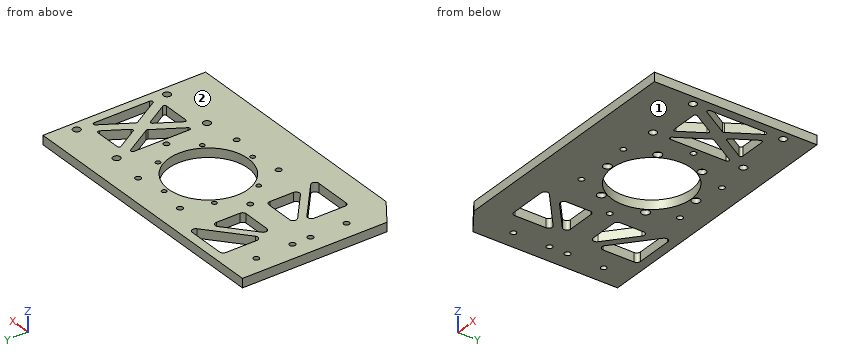
from build123d import *

# Parameters (mm, degrees)
SKETCH_1_W             = 150
SKETCH_1_H             = 80
SKETCH_1_R             = 1.3
SKETCH_1_R_2           = 22
EXTRUDE_1_DEPTH        = 5
SKETCH_3_R             = 1.55
SKETCH_3_R_2           = 1.582849294
CUT_EXTRUDE_3_DEPTH    = 12.5
CUT_EXTRUDE_5_DEPTH    = 8
FILLET_3_R             = 2
FILLET_3_OF_MIRROR_2_R = 2
EXTRUDE_4_DEPTH        = 5
FILLET_5_R             = 5
SKETCH_11_R            = 1.55
CUT_EXTRUDE_7_DEPTH    = 25
SKETCH_12_R            = 2.05
CUT_EXTRUDE_8_DEPTH    = 10
CUT_EXTRUDE_9_DEPTH    = 10
FILLET_6_R             = 1
EXTRUDE_5_DEPTH        = 5
SKETCH_16_R            = 2.25
CUT_EXTRUDE_10_DEPTH   = 2.5
CUT_EXTRUDE_START      = -10
CUT_EXTRUDE_11_DEPTH   = 10


with BuildPart() as part:
    # 草图1 → 凸台-拉伸1 (new body)
    with BuildSketch(Plane.XY):
        with Locations((-5, 0)):
            Rectangle(SKETCH_1_W, SKETCH_1_H)
        with Locations((0, -24.5)):
            Circle(SKETCH_1_R, mode=Mode.SUBTRACT)
        with Locations((-21.217622393, -12.25)):
            Circle(SKETCH_1_R, mode=Mode.SUBTRACT)
        with Locations((-21.217622393, 12.25)):
            Circle(SKETCH_1_R, mode=Mode.SUBTRACT)
        Circle(SKETCH_1_R_2, mode=Mode.SUBTRACT)
        with Locations((0, 24.5)):
            Circle(SKETCH_1_R, mode=Mode.SUBTRACT)
        with Locations((21.217622393, 12.25)):
            Circle(SKETCH_1_R, mode=Mode.SUBTRACT)
        with Locations((21.217622393, -12.25)):
            Circle(SKETCH_1_R, mode=Mode.SUBTRACT)
    extrude(amount=EXTRUDE_1_DEPTH)

    # 草图3 → 切除-拉伸3 (cut)
    with BuildSketch(Plane.XY.offset(5)):
        with Locations((-70, -25)):
            Circle(SKETCH_3_R)
        with Locations((-70, -5)):
            Circle(SKETCH_3_R_2)
        with Locations((-70, 25)):
            Circle(SKETCH_3_R)
        with Locations((-70, 5)):
            Circle(SKETCH_3_R_2)
    extrude(amount=-CUT_EXTRUDE_3_DEPTH, mode=Mode.SUBTRACT)

    # 草图4 → 切除-拉伸5 (cut)
    with BuildSketch(Plane.XY.offset(5)):
        Polygon((-58, 35), (-30, 35), (-58, 11.505210327), align=None)
        Polygon((-35, 25.582872687), (-58, 6.28358117), (-35, 6.28358117), align=None)
    cut_extrude_5 = extrude(amount=-CUT_EXTRUDE_5_DEPTH, mode=Mode.SUBTRACT)

    # 圆角3
    fillet_3_edges = [part.edges().sort_by_distance(p)[0] for p in [
        (-35, 6.28358117, 2.5),
        (-58, 6.28358117, 2.5),
        (-35, 25.582872687, 2.5),
        (-30, 35, 2.5),
        (-58, 11.505210327, 2.5),
        (-58, 35, 2.5),
    ]]
    fillet(fillet_3_edges, radius=FILLET_3_R)

    # 镜向2: 切除-拉伸5 across plane
    add(cut_extrude_5.mirror(Plane.ZX), mode=Mode.SUBTRACT)

    # 圆角3 of 镜向2
    fillet_3_of_mirror_2_edges = [part.edges().sort_by_distance(p)[0] for p in [
        (-35, -6.28358117, 2.5),
        (-58, -6.28358117, 2.5),
        (-35, -25.582872687, 2.5),
        (-30, -35, 2.5),
        (-58, -11.505210327, 2.5),
        (-58, -35, 2.5),
    ]]
    fillet(fillet_3_of_mirror_2_edges, radius=FILLET_3_OF_MIRROR_2_R)

    # 草图10 → 凸台-拉伸4 (add)
    with BuildSketch(Plane.XY.offset(5)):
        Polygon((-80, -40), (-127.053079228, -7.053079228), (-80, 40), align=None)
    extrude(amount=-EXTRUDE_4_DEPTH)

    # 圆角5
    fillet_5_edges = [part.edges().sort_by_distance(p)[0] for p in [
        (-127.053079228, -7.053079228, 2.5),
    ]]
    fillet(fillet_5_edges, radius=FILLET_5_R)

    # 草图11 → 切除-拉伸7 (cut)
    with BuildSketch(Plane.XY.offset(5)):
        with Locations((-15.75, 27.279800219)):
            Circle(SKETCH_11_R)
        with Locations((15.75, 27.279800219)):
            Circle(SKETCH_11_R)
        with Locations((31.5, 0)):
            Circle(SKETCH_11_R)
        with Locations((15.75, -27.279800219)):
            Circle(SKETCH_11_R)
        with Locations((-15.75, -27.279800219)):
            Circle(SKETCH_11_R)
        with Locations((-31.5, 0)):
            Circle(SKETCH_11_R)
    extrude(amount=-CUT_EXTRUDE_7_DEPTH, mode=Mode.SUBTRACT)

    # 草图12 → 切除-拉伸8 (cut)
    with BuildSketch(Plane.XY.offset(5)):
        with Locations((35, 25)):
            Circle(SKETCH_12_R)
        with Locations((65, 25)):
            Circle(SKETCH_12_R)
        with Locations((65, -25)):
            Circle(SKETCH_12_R)
        with Locations((35, -25)):
            Circle(SKETCH_12_R)
    extrude(amount=-CUT_EXTRUDE_8_DEPTH, mode=Mode.SUBTRACT)

    # 草图13 → 切除-拉伸9 (cut)
    with BuildSketch(Plane.XY.offset(5)):
        Polygon((35, 19), (35, -19), (46.4, 0), align=None)
        Polygon((65, -19), (53.6, 0), (65, 19), align=None)
        Polygon((41, 19), (50, 4), (59, 19), align=None)
        Polygon((50, -4), (59, -19), (41, -19), align=None)
    extrude(amount=-CUT_EXTRUDE_9_DEPTH, mode=Mode.SUBTRACT)

    # 圆角6
    fillet_6_edges = [part.edges().sort_by_distance(p)[0] for p in [
        (41, 19, 2.5),
        (59, 19, 2.5),
        (50, 4, 2.5),
        (65, 19, 2.5),
        (65, -19, 2.5),
        (53.6, 0, 2.5),
        (41, -19, 2.5),
        (50, -4, 2.5),
        (59, -19, 2.5),
        (35, 19, 2.5),
        (46.4, 0, 2.5),
        (35, -19, 2.5),
    ]]
    fillet(fillet_6_edges, radius=FILLET_6_R)

    # 草图14 → 凸台-拉伸5 (add)
    with BuildSketch(Plane.XY.offset(5)):
        Polygon((-80, -40), (-65.718519933, -50), (70, -50), (70, -40), align=None)
    extrude(amount=-EXTRUDE_5_DEPTH)

    # 草图16 → 切除-拉伸10 (cut)
    with BuildSketch(Plane(origin=(0, 0, 0), x_dir=(-1, 0, 0), z_dir=(0, 0, -1))):
        with Locations((0, 24.5)):
            Circle(SKETCH_16_R)
        with Locations((21.217622393, 12.25)):
            Circle(SKETCH_16_R)
        with Locations((21.217622393, -12.25)):
            Circle(SKETCH_16_R)
        with Locations((0, -24.5)):
            Circle(SKETCH_16_R)
        with Locations((-21.217622393, -12.25)):
            Circle(SKETCH_16_R)
        with Locations((-21.217622393, 12.25)):
            Circle(SKETCH_16_R)
    extrude(amount=-CUT_EXTRUDE_10_DEPTH, mode=Mode.SUBTRACT)

    # 草图17 → 切除-拉伸11 (cut)
    with BuildSketch(Plane.XY.offset(5).offset(CUT_EXTRUDE_START)):
        with BuildLine():
            Line((-122.839593994, -2.839593994), (-80, 40))
            Line((-80, 40), (-80, 0))
            Line((-80, 0), (-80, -40))
            Line((-80, -40), (-122.17194227, -10.470888122))
            ThreePointArc((-122.17194227, -10.470888122), (-124.285033579, -6.810906614), (-122.839593994, -2.839593994))
        make_face()
    extrude(amount=CUT_EXTRUDE_11_DEPTH, mode=Mode.SUBTRACT)


solid = part.part
Geometry check sheet. Reference: the model listing, model coordinates, mm. Face numbers are marked on the shaded views. Give positions to 0.01 mm unless a question says otherwise; leave off trailing zeros. Order: outer loops, then holes, each group sorted by start corner. A loop starts at its lowest first (then second) coordinate and runs counter-clockwise, first axis right, second up.
1) Cross-section at D-D (z = 3.35). Give the number of separate pieces and of enclosed holes in the cut face, then the cut area to 4 significant figures.
Results are:
separate pieces: 1
enclosed holes: 29
area: 10,000 mm2
2) Draft check along Z on the marked faces 1 and 2. Enter one of: released by +Z, released by -Z, zero draft, split by the parting line, or undercut.
Results are:
face 1: released by -Z
face 2: released by +Z
3) Cross-section at A-A (x = -31.5). Record the boundary of the cut face in (y, z).
Results are:
outline: (-50, 0) - (-1.55, 0) - (-1.55, 5) - (-50, 5) - close; (1.55, 0) - (40, 0) - (40, 5) - (1.55, 5) - close
4) Cross-section at B-B (x = -15.75). Record the boundary of the cut face in (y, z), then the cut area to 3 significant figures.
Results are:
outline: (-50, 0) - (-28.83, 0) - (-28.83, 5) - (-50, 5) - close; (-25.73, 0) - (-15.36, 0) - (-15.36, 5) - (-25.73, 5) - close; (15.36, 0) - (25.73, 0) - (25.73, 5) - (15.36, 5) - close; (28.83, 0) - (40, 0) - (40, 5) - (28.83, 5) - close
area: 265 mm2
5) Material ranges on probe 1 along Y at (x, z) = (0, 1.75); probe 2 along Y at (x, z) = (0, 3.4); probe 3 along X at (y, z) = (-17, 1.4), recorded low to high.
Results are:
probe 1: y = -50 to -26.75, -22.25 to -22, 22 to 22.25, 26.75 to 40
probe 2: y = -50 to -25.8, -23.2 to -22, 22 to 23.2, 25.8 to 40
probe 3: x = -80 to -58, -51.45 to -45.23, -35 to -13.96, 13.96 to 42.2, 57.8 to 70
6) Gauge pin test, flat ends, axial feed: pin 1 (6 mm diameter, centred on x = 21.22, y = -12.25, fed in from +Z); pin 2 (2.5 mm diameter, centred on x = -21.22, y = 12.25, fed in from +Z); pin 3 (4 mm diameter, centred on x = 21.22, y = -12.25, fed in from -Z). Record the tip position at first contact, or that the pin passes through.
Results are:
pin 1: stops at z = 5
pin 2: passes through
pin 3: stops at z = 2.5
7) Cross-section at C-C (x = -51). Record the boundary of the cut face in (y, z).
Results are:
outline: (-50, 0) - (-35, 0) - (-35, 5) - (-50, 5) - close; (-17.38, 0) - (-12.16, 0) - (-12.16, 5) - (-17.38, 5) - close; (-6.28, 0) - (6.28, 0) - (6.28, 5) - (-6.28, 5) - close; (12.16, 0) - (17.38, 0) - (17.38, 5) - (12.16, 5) - close; (35, 0) - (40, 0) - (40, 5) - (35, 5) - close
